Design review of the part shown in the three views and the two pictorial views. Dimensions are in mm from the part's minimum x, y and z. Coordinates: 2 decimals unless noted, no trailing zeros. Write each loop counter-clockwise with the first axis right and the second up, starting at its lowest first coordinate (ties: lowest second). Pieces come first, ordered by that corner, then holes. Notation, with made-up numbers: (-13.75, -37.5) - (-8.75, -37.5) arc R17 ccw to (-8.75, -12.5) - close; hole circle Ø9 at (71.5, 54.5). An arc over 180 degrees is marked (long way). Write each question's results on one line, items separated by ' | '.
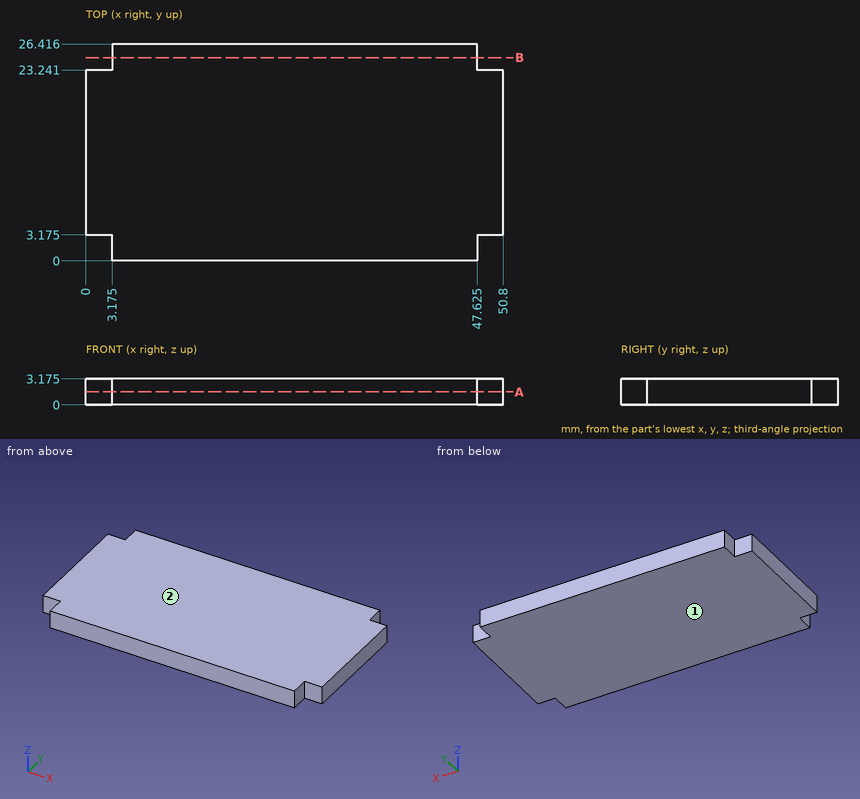
Q1. Wall thickness on line 1 along X through (y, z) = (25.25, 2.25) (3 decimals); line 2 along Y through (x, z) = (2, 2.95) (3 decimals): over which ranges is each line inside the solid? List them lowest first. Write a range as from..to.
Results found:
line 1: 3.175..47.625 | line 2: 3.175..23.241
Q2. For pin 1 (1 mm diameter, centred on x = 2, z = 1, fed in from +Y); pin 2 (1.6 mm diameter, centred on y = 25, z = 1, fed in from +X) (3 decimals); pin 3 (1 mm diameter, centred on y = 24, z = 1.5, fed in from -X) (3 decimals), all flat-tipped, find the tip position at first contact; note any pin that passes through.
Results found:
pin 1: y = 23.24 | pin 2: x = 47.625 | pin 3: x = 3.175
Q3. Take a section at A-A on z = 1.6. State the section outline as (x, y) points (3 decimals).
Results found:
outline: (0, 3.175) - (3.175, 3.175) - (3.175, 0) - (47.625, 0) - (47.625, 3.175) - (50.8, 3.175) - (50.8, 23.241) - (47.625, 23.241) - (47.625, 26.416) - (3.175, 26.416) - (3.175, 23.241) - (0, 23.241) - close
Q4. Mouldability with a two-part tool opening along Z and no side actions: class the marked faces 1 and 2 as pulls with the +Z half, pulls with the -Z half, needs draft (parallel to the pull), parting line crosses it, or undercut.
Results found:
face 1: pulls with the -Z half | face 2: pulls with the +Z half
Q5. Take a section at B-B on y = 24.75. State the section outline as (x, z) points (3 decimals), plus the area to 3 significant figures.
Results found:
outline: (3.175, 0) - (47.625, 0) - (47.625, 3.175) - (3.175, 3.175) - close | area: 141 mm2
